Read the model definition and answer for the solid it produces. Units are mm, in the model's axes. Face numbers are marked on the shaded views. A direction names the side the tool comes from. Coordinates: 2 decimals unless noted, no trailing zeros. Loops run counter-clockwise (first coordinate to the right, second up) from the corner with the lowest first, then second, coordinate; pieces in that order, holes last. Notation, with made-up numbers: (-0.5, 82.25) -> (33.5, 82.25) arc R15 cw to (33.5, 108.25) -> close; hole circle Ø3 at (0, -38). An arc over 180 degrees is marked (long way). Answer as a JSON object with one key per item and string values. Group by question number.
Q1. The part is cut by section B-B on y = 13. Write down the section's boundary in (x, z).
Q2. The part is cut by section C-C on x = 12.5. Write down the section's boundary in (y, z).
Q3. Straight lines are drawn through the part: line 1 along Y through (x, z) = (0, 15); line 2 along Z through (x, y) = (9, -5); line 3 along X through (y, z) = (-12, 13). For each, find the intervals that lie inside material, in ascending order. Write a range as [from, to].
Q4. The part is cut by section D-D on z = -13.5. Write down the section's boundary in (x, y), and give its area (3 significant figures).
Q5. For the marked faces 1 and 2, determine the directions among +Z, -Z, +X, -X, +Y, -Y from which every point of the face is accessible in a straight line to the end or side of a thin tool.
Q6. Each of these flat-tipped pins is pushed along its axis until it touches: P1, Ø5, axis at x = -5.5, z = 0.5, coming from the +Y side; P2, Ø5, axis at x = 0, y = 12.5, coming from the -Z side; P3, Ø10, axis at x = 5, z = 4.5, coming from the +Y side. Where does it stop, or does it pass through?
Q7. The part is cut by section A-A on x = 0. Write down the section's boundary in (y, z), and give its area (3 significant figures).
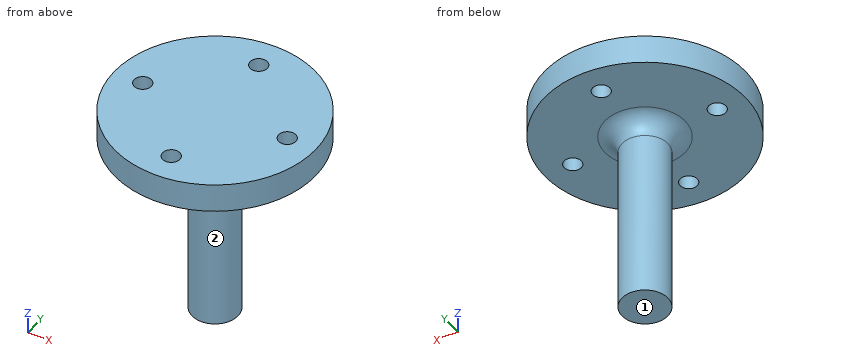
from build123d import *

# Parameters (mm, degrees)
SKETCH1_R                = 4
BOSS_EXTRUDE1_DEPTH      = 12.451061179
BOSS_EXTRUDE1_DEPTH_BACK = 20
SKETCH3_R                = 17.5
SKETCH3_R_2              = 1.5
BOSS_EXTRUDE2_DEPTH      = 5
FILLET1_R                = 3


with BuildPart() as part:
    # Sketch1 → Boss-Extrude1 (new body, two sides)
    with BuildSketch(Plane.XY) as boss_extrude1_sk:
        Circle(SKETCH1_R)
    extrude(amount=BOSS_EXTRUDE1_DEPTH)
    extrude(boss_extrude1_sk.sketch, amount=-BOSS_EXTRUDE1_DEPTH_BACK)

    # Sketch3 → Boss-Extrude2 (add)
    with BuildSketch(Plane.XY.offset(12.451061179)):
        Circle(SKETCH3_R)
        with Locations((0, 12.5)):
            Circle(SKETCH3_R_2, mode=Mode.SUBTRACT)
        with Locations((12.5, 0)):
            Circle(SKETCH3_R_2, mode=Mode.SUBTRACT)
        with Locations((0, -12.5)):
            Circle(SKETCH3_R_2, mode=Mode.SUBTRACT)
        with Locations((-12.5, 0)):
            Circle(SKETCH3_R_2, mode=Mode.SUBTRACT)
    extrude(amount=BOSS_EXTRUDE2_DEPTH)

    # Fillet1
    fillet1_edges = [part.edges().sort_by_distance(p)[0] for p in [
        (-4, 0, 12.451061179),
    ]]
    fillet(fillet1_edges, radius=FILLET1_R)


solid = part.part
Final values:
{
 "1": {"outline": "(-11.72, 12.45) -> (-1.41, 12.45) -> (-1.41, 17.45) -> (-11.72, 17.45) -> close; (1.41, 12.45) -> (11.72, 12.45) -> (11.72, 17.45) -> (1.41, 17.45) -> close"},
 "2": {"outline": "(-12.25, 12.45) -> (-1.5, 12.45) -> (-1.5, 17.45) -> (-12.25, 17.45) -> close; (1.5, 12.45) -> (12.25, 12.45) -> (12.25, 17.45) -> (1.5, 17.45) -> close"},
 "3": {"line 1": "y = [-17.5, -14], [-11, 11], [14, 17.5]", "line 2": "z = [12.45, 17.45]", "line 3": "x = [-12.74, -1.41], [1.41, 12.74]"},
 "4": {"outline": "circle Ø8 at (0, 0)", "area": "50.3 mm2"},
 "5": {"face 1": "-Z, +X, -X, +Y, -Y", "face 2": "-Z"},
 "6": {"P1": "stops at y = 2.65", "P2": "stops at z = 12.45", "P3": "stops at y = 4"},
 "7": {"outline": "(-17.5, 12.45) -> (-14, 12.45) -> (-14, 17.45) -> (-17.5, 17.45) -> close; (-11, 12.45) -> (-7, 12.45) arc R3 cw to (-4, 9.45) -> (-4, -20) -> (4, -20) -> (4, 9.45) arc R3 cw to (7, 12.45) -> (11, 12.45) -> (11, 17.45) -> (-11, 17.45) -> close; (14, 12.45) -> (17.5, 12.45) -> (17.5, 17.45) -> (14, 17.45) -> close", "area": "408 mm2"}
}
